Geometry: final body of the model. Coordinates: model frame, mm. A direction names the side the tool comes from. Round coordinates to 2 decimals unless told otherwise and drop trailing zeros. Loops run counter-clockwise (first coordinate to the right, second up) from the corner with the lowest first, then second, coordinate; pieces in that order, holes last. Notation, with made-up numbers: (14, -31) - (68, -31) arc R17 ccw to (68, -27) - close; hole circle Ø7 at (-11, 50.5). An arc over 180 degrees is marked (long way). Answer as a JSON object with one key per item and string values. Group by question number.
Item 1: First-contact query: pin 1 (1 mm diameter, centred on x = -1, y = 1, fed in from +Z); pin 2 (1.5 mm diameter, centred on x = 1.5, y = -2, fed in from -Z); pin 3 (2 mm diameter, centred on y = 1.5, z = -1.5, fed in from -X); pin 4 (4.5 mm diameter, centred on x = 0, z = 0, fed in from +Y). Flat tips, straight axial feed; report the tip coordinate or a pass-through.
Item 2: Section A-A (z = 0). Return the cut outline in (x, y).
Item 3: Line query: line 1 (Z direction, x = 0, y = -2.4); line 2 (X direction, y = 2.15, z = 0.5). Output: solid intervals per line, ascending.
Item 4: Section D-D (y = -1.7). Return the cut outline in (x, z).
Item 5: Draft query along X for faces 4 (the face through (2, -2.5, 2)), 5 (the face through (-1.73, 0.04, 7.81)), 6 (the face through (6.466, 2.303, 2.681)). Return one class per face: released by +X, released by -X, zero draft, split by the parting line, or undercut.
Item 6: Section C-C (x = -5). Return the cut outline in (y, z) (3 decimals), plus the area to 3 significant figures.
Item 7: Section B-B (x = 0). Return the cut outline in (y, z).
Item 8: Reachability of faces 1 (the face through (3, 2.1, 3)), 2 (the face through (2, 2.5, 2)), 3 (the face through (6.466, -2.303, 2.681)) from +Z, -Z, +X, -X, +Y, -Y: full face, straight path, thin tool, end or side. Return the list, or none.
```python
from build123d import *

# Parameters (mm, degrees)
SKETCH1_R                = 8
BOSS_EXTRUDE1_DEPTH      = 2.5
BOSS_EXTRUDE1_DEPTH_BACK = 2.5
SKETCH2_R                = 2.5
CUT_EXTRUDE1_DEPTH       = 6
SKETCH3_R                = 7
SKETCH3_R_2              = 3.5
CUT_EXTRUDE2_DEPTH       = 0.4


with BuildPart() as part:
    # Sketch1 → Boss-Extrude1 (new body, two sides)
    with BuildSketch(Plane(origin=(0, 0, 0), x_dir=(1, 0, 0), z_dir=(0, 1, 0))) as boss_extrude1_sk:
        Circle(SKETCH1_R)
    extrude(amount=BOSS_EXTRUDE1_DEPTH)
    extrude(boss_extrude1_sk.sketch, amount=-BOSS_EXTRUDE1_DEPTH_BACK)

    # Sketch2 → Cut-Extrude1 (cut, through all)
    with BuildSketch(Plane(origin=(0, 2.5, 0), x_dir=(1, 0, 0), z_dir=(0, 1, 0))):
        Circle(SKETCH2_R)
    extrude(amount=-CUT_EXTRUDE1_DEPTH, mode=Mode.SUBTRACT)

    # Sketch3 → Cut-Extrude2 (cut)
    with BuildSketch(Plane(origin=(0, 2.5, 0), x_dir=(1, 0, 0), z_dir=(0, 1, 0))):
        Circle(SKETCH3_R)
        Circle(SKETCH3_R_2, mode=Mode.SUBTRACT)
    cut_extrude2 = extrude(amount=-CUT_EXTRUDE2_DEPTH, mode=Mode.SUBTRACT)

    # Mirror1: Cut-Extrude2 across plane
    add(cut_extrude2.mirror(Plane.ZX), mode=Mode.SUBTRACT)


solid = part.part
```
Values:
{
 "1": {"pin 1": "stops at z = 7.98", "pin 2": "stops at z = -7.96", "pin 3": "stops at x = -7.98", "pin 4": "passes through"},
 "2": {"outline": "(-8, -2.5) - (-7, -2.5) - (-7, -2.1) - (-3.5, -2.1) - (-3.5, -2.5) - (-2.5, -2.5) - (-2.5, 2.5) - (-3.5, 2.5) - (-3.5, 2.1) - (-7, 2.1) - (-7, 2.5) - (-8, 2.5) - close; (2.5, -2.5) - (3.5, -2.5) - (3.5, -2.1) - (7, -2.1) - (7, -2.5) - (8, -2.5) - (8, 2.5) - (7, 2.5) - (7, 2.1) - (3.5, 2.1) - (3.5, 2.5) - (2.5, 2.5) - close"},
 "3": {"line 1": "z = -8 to -7, -3.5 to -2.5, 2.5 to 3.5, 7 to 8", "line 2": "x = -7.98 to -6.98, -3.46 to -2.45, 2.45 to 3.46, 6.98 to 7.98"},
 "4": {"outline": "circle Ø16 at (0, 0); hole circle Ø5 at (0, 0)"},
 "5": {"face 4": "zero draft", "face 5": "split by the parting line", "face 6": "undercut"},
 "6": {"outline": "(-2.5, -6.245) - (2.5, -6.245) - (2.5, -4.899) - (2.1, -4.899) - (2.1, 4.899) - (2.5, 4.899) - (2.5, 6.245) - (-2.5, 6.245) - (-2.5, 4.899) - (-2.1, 4.899) - (-2.1, -4.899) - (-2.5, -4.899) - close", "area": "54.6 mm^2"},
 "7": {"outline": "(-2.5, -8) - (2.5, -8) - (2.5, -7) - (2.1, -7) - (2.1, -3.5) - (2.5, -3.5) - (2.5, -2.5) - (-2.5, -2.5) - (-2.5, -3.5) - (-2.1, -3.5) - (-2.1, -7) - (-2.5, -7) - close; (-2.5, 2.5) - (2.5, 2.5) - (2.5, 3.5) - (2.1, 3.5) - (2.1, 7) - (2.5, 7) - (2.5, 8) - (-2.5, 8) - (-2.5, 7) - (-2.1, 7) - (-2.1, 3.5) - (-2.5, 3.5) - close"},
 "8": {"face 1": "+Y", "face 2": "+Z, -Z, +X, -X, +Y", "face 3": "-Y"}
}
